Autodesk Inventor part; units mm, degrees
ref_plane "YZ Plane" through (0, 0, 0) normal (1, 0, 0) x (0, 1, 0)
ref_plane "XZ Plane" through (0, 0, 0) normal (0, 1, 0) x (-1, 0, 0)
ref_plane "XY Plane" through (0, 0, 0) normal (0, 0, 1) x (1, 0, 0)
sketch "Sketch1" plane through (0, 0, 0) normal (0, 0, 1) x (1, 0, 0)
  circle A0 centre (0, 0) radius 65
  circle A1 centre (0, 0) radius 6
  dimension "d0" = 130
  dimension "d3" = 12
extrude "Extrusion1" add sketch "Sketch1" along normal blind 15 contours A0 | A1
sketch "Sketch2" plane through (0, 0, 15) normal (0, 0, 1) x (1, 0, 0)
  circle A0 centre (0, 0) radius 6
  dimension "d4" = 12
extrude "Extrusion2" cut sketch "Sketch2" against normal blind 15
sketch "Sketch3" plane through (0, 0, 15) normal (0, 0, 1) x (1, 0, 0)
  circle A0 centre (50, 0) radius 5
  circle A1 centre (-50, 0) radius 5
  point P0 (0, 0)
  dimension "d7" = 10
  dimension "d8" = 10
extrude "Extrusion3" cut sketch "Sketch3" against normal blind 15
properties part number "doner_taban"
Part model, mm, in its own coordinate system. Round coordinates to 2 decimals unless told otherwise and drop trailing zeros. Write each loop counter-clockwise with the first axis right and the second up, starting at its lowest first coordinate (ties: lowest second). Pieces come first, ordered by that corner, then holes. Notation, with made-up numbers: (19, 30.5) -> (51, 30.5) arc R35 ccw to (51, 65.5) -> close; hole circle Ø5 at (84.5, 44.5). An arc over 180 degrees is marked (long way). Return JSON: item names as keys, results as strings. Group by question number.
Q1. Saw through at A-A on x = 0. Write the cut outline in (y, z), plus the area to 3 significant figures.
Q2. Probe L1, parallel to X at y = -1.5, z = 11; L2, parallel to Y at x = 0, z = 5; L3, parallel to Y at x = -49.5, z = 7.5. List the from-to ranges inside material, lowest first. Write a range as [from, to].
Q3. Saw through at D-D on x = -50. Write the cut outline in (y, z), plus the area to 3 significant figures.
Q4. Saw through at C-C on z = 1.5. Write the cut outline in (x, y).
Q5. Saw through at B-B on y = 0. Write the cut outline in (x, z), plus the area to 3 significant figures.
Q6. Pin check, flat tips, straight feed: pin 1 (3 mm diameter, centred on x = -7, z = 10, fed in from -Y); pin 2 (1.5 mm diameter, centred on x = 29, y = -49.5, fed in from -Z); pin 3 (1 mm diameter, centred on x = 27, z = 6, fed in from -Y); pin 4 (2 mm diameter, centred on x = 45, z = 12, fed in from +Y). Stop position of each tip, or through.
Q7. Mould opens along X. For faces 1 (the cylindrical face through (62, -19.52, 7.4)), 2 (the cylindrical face through (-6, 0, 8)), 3 (the cylindrical face through (45, 0, 8)), 4 (the flat face through (14, 1, 15)) say: pulls with the +X half, pulls with the -X half, needs draft (parallel to the pull), parting line crosses it, or undercut.
Answer:
{
 "1": {"outline": "(-65, 0) -> (-6, 0) -> (-6, 15) -> (-65, 15) -> close; (6, 0) -> (65, 0) -> (65, 15) -> (6, 15) -> close", "area": "1,770 mm2"},
 "2": {"L1": "[-64.98, -54.77], [-45.23, -5.81], [5.81, 45.23], [54.77, 64.98]", "L2": "[-65, -6], [6, 65]", "L3": "[-42.13, -4.97], [4.97, 42.13]"},
 "3": {"outline": "(-41.53, 0) -> (-5, 0) -> (-5, 15) -> (-41.53, 15) -> close; (5, 0) -> (41.53, 0) -> (41.53, 15) -> (5, 15) -> close", "area": "1,100 mm2"},
 "4": {"outline": "circle Ø130 at (0, 0); hole circle Ø10 at (-50, 0); hole circle Ø12 at (0, 0); hole circle Ø10 at (50, 0)"},
 "5": {"outline": "(-65, 0) -> (-55, 0) -> (-55, 15) -> (-65, 15) -> close; (-45, 0) -> (-6, 0) -> (-6, 15) -> (-45, 15) -> close; (6, 0) -> (45, 0) -> (45, 15) -> (6, 15) -> close; (55, 0) -> (65, 0) -> (65, 15) -> (55, 15) -> close", "area": "1,470 mm2"},
 "6": {"pin 1": "y = -64.77", "pin 2": "z = 0", "pin 3": "y = -59.35", "pin 4": "y = 47.84"},
 "7": {"face 1": "parting line crosses it", "face 2": "undercut", "face 3": "undercut", "face 4": "needs draft"}
}
